Geometry: final body of the model. Coordinates: model frame, mm. Give positions to 0.01 mm unless a question says otherwise; leave off trailing zeros. Write each loop counter-clockwise with the first axis right and the second up, starting at its lowest first coordinate (ties: lowest second). Pieces come first, ordered by that corner, then holes. Notation, with made-up numbers: M 81.5,-10.5 L 102.5,-10.5 A22 cw 102.5,0.5 Z; hole C 3.5,-33 d1. An arc over 180 degrees is marked long. Answer as a JSON object with one key per item and string values.
Autodesk Inventor part; units mm, degrees
ref_plane "YZ Plane" through (0, 0, 0) normal (1, 0, 0) x (0, 1, 0)
ref_plane "XZ Plane" through (0, 0, 0) normal (0, 1, 0) x (-1, 0, 0)
ref_plane "XY Plane" through (0, 0, 0) normal (0, 0, 1) x (1, 0, 0)
sketch "Sketch1" plane through (0, 0, 0) normal (0, 1, 0) x (-1, 0, 0)
  line L0 (0, 0) -> (42.3, 0)
  line L1 (42.3, 0) -> (42.3, -42.3)
  line L2 (42.3, -42.3) -> (0, -42.3)
  line L3 (0, -42.3) -> (0, 0)
  dimension "d0" = 42.3
extrude "Extrusion1" add sketch "Sketch1" along normal blind 4
sketch "Sketch2" plane through (0, 4, 0) normal (0, 1, 0) x (1, 0, 0)
  line L0 (0, 42.3) -> (-42.3, 42.3)
  line L1 (-42.3, 42.3) -> (-42.3, 0)
  circle A0 centre (-36.65, 5.65) radius 1.5
  circle A1 centre (-5.65, 5.65) radius 1.5
  circle A2 centre (-36.65, 36.65) radius 1.5
  circle A3 centre (-5.65, 36.65) radius 1.5
  dimension "d3" = 3
  dimension "d5" = 31
  dimension "d6" = 31
  dimension "d7" = 5.65
  dimension "d8" = 5.65
extrude "Extrusion2" cut sketch "Sketch2" against normal up to next
sketch "Sketch3" plane through (0, 4, 0) normal (0, 1, 0) x (1, 0, 0)
  line L0 (-42.3, 0) -> (0, 0)
  line L1 (-42.3, 42.3) -> (-42.3, 0)
  circle A0 centre (-21.15, 21.15) radius 12
  dimension "d11" = 24
  dimension "d12" = 21.15
  dimension "d13" = 21.15
extrude "Extrusion3" cut sketch "Sketch3" against normal up to next
properties part number "ZMotorMount"
1) Cut plane A-A on x = -36.65. Return loops of the section in (y, z), and give its area (3 significant figures).
Geometry check:
{"outline": "M 0,-42.3 L 4,-42.3 L 4,-38.15 L 0,-38.15 Z; M 0,-35.15 L 4,-35.15 L 4,-7.15 L 0,-7.15 Z; M 0,-4.15 L 4,-4.15 L 4,0 L 0,0 Z", "area": "145 mm2"}
2) Line query: line 1 (Z direction, x = -5.65, y = 2.35); line 2 (X direction, y = 2.4, z = -21.15). Output: solid intervals per line, ascending. Write a range as from..to.
Geometry check:
{"line 1": "z = -42.3..-38.15, -35.15..-7.15, -4.15..0", "line 2": "x = -42.3..-33.15, -9.15..0"}
3) Cut plane D-D on x = -21.15. Return loops of the section in (y, z), and give its area (3 significant figures).
Geometry check:
{"outline": "M 0,-42.3 L 4,-42.3 L 4,-33.15 L 0,-33.15 Z; M 0,-9.15 L 4,-9.15 L 4,0 L 0,0 Z", "area": "73.2 mm2"}
4) Cut plane C-C on z = -5.65. Return loops of the section in (x, y), and give its area (3 significant figures).
Geometry check:
{"outline": "M -42.3,0 L -38.15,0 L -38.15,4 L -42.3,4 Z; M -35.15,0 L -7.15,0 L -7.15,4 L -35.15,4 Z; M -4.15,0 L 0,0 L 0,4 L -4.15,4 Z", "area": "145 mm2"}
5) Pull-direction query (Z, two-part tool) for faces 1 (the flat face through (0, 2, -21)), 2 (the flat face through (-21, 2, -42.3)), 3 (the cylindrical face through (-30.673, 2.028, -13.848)); classes: pulls with the +Z half, pulls with the -Z half, needs draft (parallel to the pull), parting line crosses it, or undercut.
Geometry check:
{"face 1": "needs draft", "face 2": "pulls with the -Z half", "face 3": "undercut"}
6) Cut plane B-B on y = 2.05. Return loops of the section in (x, z), and give its area (3 significant figures).
Geometry check:
{"outline": "M -42.3,-42.3 L 0,-42.3 L 0,0 L -42.3,0 Z; hole C -36.65,-36.65 d3; hole C -36.65,-5.65 d3; hole C -21.15,-21.15 d24; hole C -5.65,-36.65 d3; hole C -5.65,-5.65 d3", "area": "1,310 mm2"}
